For this review, take the finished solid that the model builds, in its own axes (mm). A direction names the side the tool comes from. Coordinates: 2 decimals unless noted, no trailing zeros. Loops run counter-clockwise (first coordinate to the right, second up) from the corner with the lowest first, then second, coordinate; pieces in that order, holes last. Notation, with made-up numbers: (-11, -22) -> (-7, -22) arc R28 ccw to (-7, 6) -> close; hole circle Ø3 at (51.25, 63.5). An arc over 180 degrees is marked (long way). One line per item, written item: value.
from build123d import *

# Parameters (mm, degrees)
F0_W     = 30
F0_H     = 43
F1_DEPTH = 2
F3_DEPTH = 2
F4_W     = 30
F4_H     = 43
F5_DEPTH = 2


with BuildPart() as f1:
    # F0 (on Top) → F1 (new body)
    with BuildSketch(Plane.XY):
        Rectangle(F0_W, F0_H)
    extrude(amount=F1_DEPTH)

    # F2 (on face) → F3 (join)
    with BuildSketch(Plane.XY.offset(2)):
        Polygon((-13.862556, -20.510625), (-13.862556, 21.5), (-15, 21.5), (-15, -21.5), (15, -21.5), (15, 21.5), (13.922185, 21.5), (13.922185, -20.510625), align=None)
    extrude(amount=F3_DEPTH)

    # F4 (on face) → F5 (join)
    with BuildSketch(Plane.XY.offset(4)):
        Rectangle(F4_W, F4_H)
    extrude(amount=F5_DEPTH)


solid = f1.part
1. Take a section at C-C, the plane x = 2. Give the boundary of the cut face in (y, z).
Return value:
outline: (-21.5, 0) -> (21.5, 0) -> (21.5, 2) -> (-20.51, 2) -> (-20.51, 4) -> (21.5, 4) -> (21.5, 6) -> (-21.5, 6) -> close
2. To check wall thickness, follow probe 1 along Z at (x, y) = (-11.5, -9); probe 2 along X at (y, z) = (-10.5, 3.35); probe 3 along Y at (x, z) = (13.75, 3.05). State the ranges of each line that lie inside material, in increasing order. Write a range as from..to.
Return value:
probe 1: z = 0..2, 4..6
probe 2: x = -15..-13.86, 13.92..15
probe 3: y = -21.5..-20.51
3. Take a section at A-A, the plane y = 13. Give the boundary of the cut face in (x, z).
Return value:
outline: (-15, 0) -> (15, 0) -> (15, 6) -> (-15, 6) -> close; hole (-13.86, 2) -> (13.92, 2) -> (13.92, 4) -> (-13.86, 4) -> close
4. The part is to be moulded in two halves that separate along X. For faces 1 (the flat face through (15, 0, 3)), 2 (the flat face through (0, -21.5, 3)), 3 (the flat face through (0, -20.511, 3)), say which applies: pulls with the +X half, pulls with the -X half, needs draft (parallel to the pull), parting line crosses it, or undercut.
Return value:
face 1: pulls with the +X half
face 2: needs draft
face 3: undercut
5. For faces 4 (the flat face through (0, 0, 0)), 5 (the flat face through (0, 1, 4)), list the 3-axis set-ups (+Z, -Z, +X, -X, +Y, -Y) from which the entire face can be reached by the end or side of a thin tool; tool diameter is ignored.
Return value:
face 4: -Z, +X, -X, +Y, -Y
face 5: +Y
6. Take a section at B-B, the plane z = 2.8. Give the boundary of the cut face in (x, y).
Return value:
outline: (-15, -21.5) -> (15, -21.5) -> (15, 21.5) -> (13.92, 21.5) -> (13.92, -20.51) -> (-13.86, -20.51) -> (-13.86, 21.5) -> (-15, 21.5) -> close
